```python
from build123d import *

# Parameters (mm, degrees)
SKIZZE1_W                                            = 180
SKIZZE1_H                                            = 65
AUFSATZ_LINEAR_AUSTRAGEN1_DEPTH                      = 5
STIRNSENKUNG_F_R_M3_ZYLINDERSCHRAUBE_MIT_D           = 3.6
STIRNSENKUNG_F_R_M3_ZYLINDERSCHRAUBE_MIT_DEPTH       = 9.1
STIRNSENKUNG_F_R_M3_ZYLINDERSCHRAUBE_MIT_CBORE_D     = 6.5
STIRNSENKUNG_F_R_M3_ZYLINDERSCHRAUBE_MIT_CBORE_DEPTH = 3.4
STIRNSENKUNG_F_R_M3_ZYLINDERSCHRAUBE_MIT_TIP         = 1.081549114
SCHNITT_LINEAR_AUSTRAGEN1_DEPTH                      = 66


with BuildPart() as part:
    # Skizze1 → Aufsatz-Linear austragen1 (new body)
    with BuildSketch(Plane.XY):
        Rectangle(SKIZZE1_W, SKIZZE1_H)
    extrude(amount=AUFSATZ_LINEAR_AUSTRAGEN1_DEPTH)

    # Stirnsenkung für M3 Zylinderschraube mit Innensechskant1
    with Locations(Plane.XY.offset(5)):
        with Locations((-84, 0), (84, 0)):
            CounterBoreHole(STIRNSENKUNG_F_R_M3_ZYLINDERSCHRAUBE_MIT_D / 2, STIRNSENKUNG_F_R_M3_ZYLINDERSCHRAUBE_MIT_CBORE_D / 2, STIRNSENKUNG_F_R_M3_ZYLINDERSCHRAUBE_MIT_CBORE_DEPTH, depth=STIRNSENKUNG_F_R_M3_ZYLINDERSCHRAUBE_MIT_DEPTH)
            with Locations((0, 0, -(STIRNSENKUNG_F_R_M3_ZYLINDERSCHRAUBE_MIT_DEPTH + STIRNSENKUNG_F_R_M3_ZYLINDERSCHRAUBE_MIT_TIP / 2))):  # 118° drill point
                Cone(0, STIRNSENKUNG_F_R_M3_ZYLINDERSCHRAUBE_MIT_D / 2, STIRNSENKUNG_F_R_M3_ZYLINDERSCHRAUBE_MIT_TIP, mode=Mode.SUBTRACT)

    # Skizze6 → Schnitt-Linear austragen1 (cut, through all)
    with BuildSketch(Plane(origin=(0, 32.5, 0), x_dir=(1, 0, 0), z_dir=(0, 1, 0))):
        with BuildLine():
            Line((-90, -5), (-90, 5))
            ThreePointArc((-90, 5), (-87.071067812, -2.071067812), (-80, -5))
            Line((-80, -5), (-90, -5))
        make_face()
        with BuildLine():
            Line((80, -5), (90, -5))
            Line((90, -5), (90, 5))
            ThreePointArc((90, 5), (87.071067812, -2.071067812), (80, -5))
        make_face()
    extrude(amount=-SCHNITT_LINEAR_AUSTRAGEN1_DEPTH, mode=Mode.SUBTRACT)


solid = part.part
```
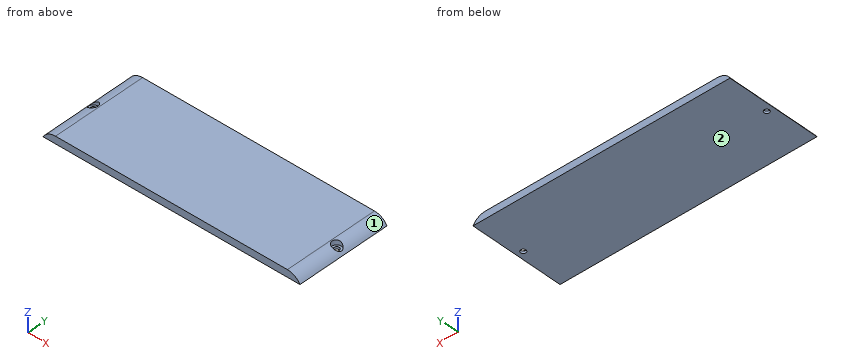
CAD build for the part. Positions are in the model's coordinates, mm. Face numbers are marked on the shaded views. Coordinates: 2 decimals unless noted, no trailing zeros. Write each loop counter-clockwise with the first axis right and the second up, starting at its lowest first coordinate (ties: lowest second). Pieces come first, ordered by that corner, then holes.
(1) Flat gauge pins, fed straight in: pin 1 (4 mm diameter, centred on x = 84, y = 0, fed in from +Z); pin 2 (3 mm diameter, centred on x = 84, y = 0, fed in from +Z); pin 3 (1 mm diameter, centred on y = -20.5, z = 3, fed in from +X). Where does each tip first touch, or does it go through?
(2) Cut at D-D, the plane y = 28.5. List the corners of the cut face in (x, z), and give its area (3 significant figures).
(3) Drill centre lines: probe 1 along Y at (x, z) = (-84, 3.8); probe 2 along Y at (x, z) = (84, 0.6); probe 3 along X at (y, z) = (15, 3.15). Where is each one in solid material? Low to high.
(4) Cut at A-A, the plane y = 0. List the corners of the cut face in (x, z).
(5) Cut at B-B, the plane x = -84. List the corners of the cut face in (y, z).
(6) Two-plate mould, pull along Z, no slides. Class the marked faces 1 and 2: +Z half, -Z half, draft (parallel to the pull), parting line (faces both ways), or undercut.
(7) Cut at C-C, the plane z = 4.05. List the corners of the cut face in (x, y), and give its area (3 significant figures).
Geometry says:
1. pin 1: stops at z = 1.6
1. pin 2: passes through
1. pin 3: stops at x = 86.61
2. outline: (-88.66, 0) - (88.66, 0) arc R10 ccw to (80, 5) - (-80, 5) arc R10 ccw to start
2. area: 861 mm2
3. probe 1: y = -32.5 to -3.25, 3.25 to 32.5
3. probe 2: y = -32.5 to -1.8, 1.8 to 32.5
3. probe 3: x = -85.79 to 85.79
4. outline: (-88.66, 0) - (-85.8, 0) - (-85.8, 1.6) - (-87.25, 1.6) - (-87.25, 1.89) arc R10 ccw to start; (-82.2, 0) - (82.2, 0) - (82.2, 1.6) - (80.75, 1.6) - (80.75, 4.97) arc R10 ccw to (80, 5) - (-80, 5) arc R10 ccw to (-80.75, 4.97) - (-80.75, 1.6) - (-82.2, 1.6) - close; (85.8, 0) - (88.66, 0) arc R10 ccw to (87.25, 1.89) - (87.25, 1.6) - (85.8, 1.6) - close
5. outline: (-32.5, 0) - (-1.8, 0) - (-1.8, 1.6) - (-3.25, 1.6) - (-3.25, 4.17) - (-32.5, 4.17) - close; (1.8, 0) - (32.5, 0) - (32.5, 4.17) - (3.25, 4.17) - (3.25, 1.6) - (1.8, 1.6) - close
6. face 1: +Z half
6. face 2: -Z half
7. outline: (-84.25, -32.5) - (84.25, -32.5) - (84.25, -3.24) arc R3.25 cw (long way) to (84.25, 3.24) - (84.25, 32.5) - (-84.25, 32.5) - (-84.25, 3.24) arc R3.25 cw (long way) to (-84.25, -3.24) - close
7. area: 10,900 mm2
